Work out the finished part from the listing and answer in its coordinate system (mm). A direction names the side the tool comes from. Give positions to 0.01 mm unless a question says otherwise; leave off trailing zeros. Loops run counter-clockwise (first coordinate to the right, second up) from the corner with the lowest first, then second, coordinate; pieces in that order, holes last.
Autodesk Fusion 360 part; units mm, degrees
sketch "Esquisse1" plane through (0, 0, 0) normal (0, 0, 1) x (1, 0, 0)
  line L0 (0, 25) -> (36, 25)
  line L1 (36, 25) -> (36, 0)
  line L2 (36, 0) -> (0, 0)
  line L3 (0, 0) -> (0, 25)
  line L4 (18, -4.4176) -> (18, 55.8936)
  circle A0 centre (10.25, 20) radius 1.075
  circle A1 centre (18, 20) radius 1.075
  line L5 (-6.2165, 12.5) -> (42, 12.5)
  circle A2 centre (9.9834, 12.5) radius 1.075
  circle A3 centre (25.75, 20) radius 1.075
  circle A4 centre (18, 20) radius 1.075
  circle A5 centre (26.0166, 12.5) radius 1.075
  circle A6 centre (10.25, 5) radius 1.075
  circle A7 centre (18, 5) radius 1.075
  circle A8 centre (25.75, 5) radius 1.075
  circle A9 centre (18, 12.5) radius 10
  circle A10 centre (18, 12.5) radius 1.75
  circle A11 centre (25.75, 20) radius 1.75
  circle A12 centre (18, 20) radius 1.75
  circle A13 centre (26.0166, 12.5) radius 1.75
  circle A14 centre (25.75, 5) radius 1.75
  circle A15 centre (18, 5) radius 1.75
  circle A16 centre (26.0166, 12.5) radius 1.75
  circle A17 centre (10.25, 20) radius 1.75
  circle A18 centre (9.9834, 12.5) radius 1.75
  circle A19 centre (10.25, 5) radius 1.75
  circle A20 centre (18, 12.5) radius 3
  point P0 (18, 12.5)
  dimension "d1" = 36
  dimension "d2" = 25
  dimension "d3" = 12.5
  dimension "d4" = 18
  dimension "d5" = 2.15
  dimension "d6" = 2.15
  dimension "d7" = 7.75
  dimension "d10" = 2.15
  dimension "d11" = 7.5
  dimension "d12" = 5
  dimension "d13" = 5
  dimension "d16" = 20
  dimension "d21" = 3.5
  dimension "d26" = 3.5
  dimension "d27" = 3.5
  dimension "d28" = 3.5
  dimension "d32" = 6
extrude "Extrusion4" add sketch "Esquisse1" along normal blind 1 contours L0 L3 L4 L5 A9 A17 | L0 L1 L4 L5 A9 A11 | L2 L3 L4 L5 A9 A19 | L1 L2 L4 L5 A9 A14 | A3 A9 A11 | A0 A9 A17 | A6 A9 A19 | A8 A9 A14 picked at (24.3887, 20.4618) picked at (11.6014, 20.4841) picked at (11.6014, 4.5159) picked at (24.3887, 4.5382)
extrude "Extrusion5" add sketch "Esquisse1" along normal blind 4.9 contours L4 L5 A9 A11 A12 A13 A16 A20 | L4 L5 A9 A12 A17 A18 A20 | L4 L5 A9 A15 A18 A19 A20 | L4 A1 A4 A12 | L4 A1 A4 A12 | A3 A9 A11 | A0 A9 A17 | L5 A2 A18 | L5 A2 A18 | A6 A9 A19 | L4 L5 A9 A13 A14 A15 A16 A20 | L5 A5 A13 A16 | L5 A5 A13 A16 | A8 A9 A14 | L4 L5 A10 A20 | L4 L5 A10 A20 | L4 A7 A15 | L4 A7 A15 | L4 L5 A10 A20 | L4 L5 A10 A20 picked at (25.5724, 18.6548) picked at (10.4124, 18.6517) picked at (10.4124, 6.3483) picked at (24.3997, 5.1334)
extrude "Extrusion6" cut sketch "Esquisse1" along normal blind 5 from surface at 1 contours L4 A1 A4 A12 | L4 A1 A4 A12 | A3 A9 A11 | A3 A9 A11 | A0 A9 A17 | A0 A9 A17 | L5 A2 A18 | L5 A2 A18 | A6 A9 A19 | A6 A9 A19 | L5 A5 A13 A16 | L5 A5 A13 A16 | A8 A9 A14 | A8 A9 A14 | L4 A7 A15 | L4 A7 A15
extrude "Extrusion8" cut sketch "Esquisse1" along normal blind 3.9 contours L4 L5 A10 A20 | L4 L5 A10 A20 | L4 L5 A10 A20 | L4 L5 A10 A20
extrude "Extrusion7" [suppressed]
Item 1: For faces 1 (the face through (8.91, 12.45, 0.49)), 2 (the face through (11.49, 6.235, 2.923)), 3 (the face through (28, 12.6, 2.9)), determine the directions among +Z, -Z, +X, -X, +Y, -Y from which every point of the face is accessible in a straight line to the end or side of a thin tool.
Item 2: Consider line 1 (Y direction, x = 18, z = 1.85); line 2 (X direction, y = 20, z = 3.6); line 3 (Y direction, x = 18, z = 4.25). Determine where each line is inside the solid, lowest interval first.
Item 3: Flat-ended cylindrical pins translate along their axes: pin 1 Ø2 at (y, z) = (4.5, 3.5) entering from +X; pin 2 Ø1 at (x, y) = (10.5, 13) entering from +Z. Find the tip coordinate at first contact, or state that the pin passes through.
Item 4: Find section D-D, the plane y = 19.5. Write down the section's boundary in (x, z).
Item 5: Find section C-C, the plane x = 3. Write down the section's boundary in (y, z), plus the area to 3 significant figures.
Item 6: Determine the mould class of faces 4 (the face through (0, 12.3, 0.5)), 5 (the face through (11.525, 18.801, 2.923)), 6 (the face through (17.9, 22.5, 2.9)) for opening direction Y: released by +Y, released by -Y, zero draft, split by the parting line, or undercut.
Item 7: Find section A-A, the plane x = 18. Give the number of separate pieces and of enclosed holes in the cut face, plus the area to 3 significant figures.
Ans:
1. face 1: +Z, -Z
1. face 2: +Z
1. face 3: +Z, +X
2. line 1: y = 2.5 to 3.25, 6.75 to 9.5, 15.5 to 18.25, 21.75 to 22.5
2. line 2: x = 12 to 16.25, 19.75 to 24
2. line 3: y = 2.5 to 3.25, 6.75 to 10.75, 14.25 to 18.25, 21.75 to 22.5
3. pin 1: stops at x = 24.07
3. pin 2: stops at z = 1
4. outline: (0, 0) - (9.3, 0) - (9.3, 1) - (0, 1) - close; (11.2, 0) - (17.05, 0) - (17.05, 1) - (16.32, 1) - (16.32, 4.9) - (11.93, 4.9) - (11.93, 1) - (11.2, 1) - close; (18.95, 0) - (24.8, 0) - (24.8, 1) - (24.07, 1) - (24.07, 4.9) - (19.68, 4.9) - (19.68, 1) - (18.95, 1) - close; (26.7, 0) - (36, 0) - (36, 1) - (26.7, 1) - close
5. outline: (0, 0) - (25, 0) - (25, 1) - (0, 1) - close
5. area: 25.0 mm2
6. face 4: zero draft
6. face 5: undercut
6. face 6: released by +Y
7. separate pieces: 4
7. enclosed holes: 0
7. area: 44.5 mm2
